```python
from build123d import *

# Parameters (mm, degrees)
SKETCH_1_R          = 8
SKETCH_1_R_2        = 4
EXTRUDE_1_DEPTH     = 7
SKETCH_2_R          = 3
EXTRUDE_2_DEPTH     = 9.5
SKETCH_5_R          = 4
CUT_EXTRUDE_1_DEPTH = 9.5
SKETCH_6_R          = 2
EXTRUDE_3_DEPTH     = 6.5
SKETCH_7_R          = 5.5
CUT_EXTRUDE_2_DEPTH = 2.5


with BuildPart() as part:
    # 草图1 → 凸台-拉伸1 (new body)
    with BuildSketch(Plane(origin=(0, 0, 0), x_dir=(1, 0, 0), z_dir=(0, 1, 0))):
        Circle(SKETCH_1_R)
        Circle(SKETCH_1_R_2, mode=Mode.SUBTRACT)
    extrude(amount=EXTRUDE_1_DEPTH)

    # 草图2 → 凸台-拉伸2 (add)
    with BuildSketch(Plane.XY):
        with Locations((0, 3.5)):
            Circle(SKETCH_2_R)
    extrude(amount=EXTRUDE_2_DEPTH)

    # 草图5 → 切除-拉伸1 (cut)
    with BuildSketch(Plane(origin=(0, 7, 0), x_dir=(1, 0, 0), z_dir=(0, 1, 0))):
        Circle(SKETCH_5_R)
    extrude(amount=-CUT_EXTRUDE_1_DEPTH, mode=Mode.SUBTRACT)

    # 草图6 → 凸台-拉伸3 (add)
    with BuildSketch(Plane.XY.offset(9.5)):
        with Locations((0, 3.5)):
            Circle(SKETCH_6_R)
    extrude(amount=EXTRUDE_3_DEPTH)

    # 草图7 → 切除-拉伸2 (cut)
    with BuildSketch(Plane(origin=(0, 7, 0), x_dir=(1, 0, 0), z_dir=(0, 1, 0))):
        Circle(SKETCH_7_R)
    extrude(amount=-CUT_EXTRUDE_2_DEPTH, mode=Mode.SUBTRACT)


solid = part.part
```
Input: part model. Units: mm. Frame: model coordinates. A direction names the side the tool comes from. Coordinates: 2 decimals unless noted, no trailing zeros. Loops run counter-clockwise (first coordinate to the right, second up) from the corner with the lowest first, then second, coordinate; pieces in that order, holes last. Notation, with made-up numbers: (71, 5) - (129, 5) arc R15 ccw to (129, 24) - close; hole circle Ø2 at (22.5, 84). An arc over 180 degrees is marked (long way). Answer in a Markdown table with one row per item.
(1) Cut plane D-D on z = -4.25. Output: boundary loops of the cut face in (x, y).
Model answer:
| item | result |
|---|---|
| outline | (-6.78, 0) - (6.78, 0) - (6.78, 7) - (3.49, 7) - (3.49, 4.5) - (-3.49, 4.5) - (-3.49, 7) - (-6.78, 7) - close |
(2) Cut plane A-A on z = 0. Output: boundary loops of the cut face in (x, y).
Model answer:
| item | result |
|---|---|
| outline | (-8, 0) - (-4, 0) - (-4, 4.5) - (-5.5, 4.5) - (-5.5, 7) - (-8, 7) - close; (4, 0) - (8, 0) - (8, 7) - (5.5, 7) - (5.5, 4.5) - (4, 4.5) - close |
(3) Cut plane C-C on y = 3.5. Output: boundary loops of the cut face in (x, z).
Model answer:
| item | result |
|---|---|
| outline | (-3, 7.42) arc R8 ccw (long way) to (3, 7.42) - (3, 9.5) - (2, 9.5) - (2, 16) - (-2, 16) - (-2, 9.5) - (-3, 9.5) - close; hole circle Ø8 at (0, 0) |
(4) Set-up query: faces 4 (the face through (1.384, 0.838, 8.675)), 5 (the face through (-4, 4.5, 2)), 6 (the face through (0, 4, 16)). Return all of +Z, -Z, +X, -X, +Y, -Y with unobstructed straight access to the full face (end or side cutting, diameter ignored); none if empty.
Model answer:
| item | result |
|---|---|
| face 4 | +Z |
| face 5 | +Y |
| face 6 | +Z, +X, -X, +Y, -Y |
(5) Mould query, pull axis X, two halves, no side actions, for faces 1 (the face through (1.7, 7, -5.4)), 2 (the face through (-1.19, 5.77, 5.37)), 3 (the face through (4.301, 3.451, -6.746)). Classes: pulls with the +X half, pulls with the -X half, needs draft (parallel to the pull), parting line crosses it, or undercut.
Model answer:
| item | result |
|---|---|
| face 1 | needs draft |
| face 2 | undercut |
| face 3 | parting line crosses it |
(6) Material intervals for L1, parallel to X at y = 5.25, z = 0; L2, parallel to X at y = 1.75, z = 0; L3, parallel to Z at x = 0, y = 1.35, sorted ascending. Write a range as from..to.
Model answer:
| item | result |
|---|---|
| L1 | x = -8..-5.5, 5.5..8 |
| L2 | x = -8..-4, 4..8 |
| L3 | z = -8..-4, 4..9.5 |
(7) Cut plane B-B on x = 0. Output: boundary loops of the cut face in (y, z), plus the area to 3 significant figures.
Model answer:
| item | result |
|---|---|
| outline | (0, -8) - (7, -8) - (7, -5.5) - (4.5, -5.5) - (4.5, -4) - (0, -4) - close; (0, 4) - (4.5, 4) - (4.5, 5.5) - (7, 5.5) - (7, 8) - (6.5, 8) - (6.5, 9.5) - (5.5, 9.5) - (5.5, 16) - (1.5, 16) - (1.5, 9.5) - (0.5, 9.5) - (0.5, 8) - (0, 8) - close |
| area | 83.5 mm² |
(8) Pin query (flat end, axial travel): P1, Ø3.5, axis at x = 0, z = 0.5, coming from the +Y side; P2, Ø2, axis at y = 4, z = 4.5, coming from the +X side; P3, Ø9, axis at x = 0, z = 0, coming from the +Y side; P4, Ø2, axis at x = -3.5, y = 3.5, coming from the -Z side. Return the tip coordinate at first contact, or that it passes through.
Model answer:
| item | result |
|---|---|
| P1 | passes through |
| P2 | stops at x = 7.19 |
| P3 | stops at y = 4.5 |
| P4 | stops at z = -7.6 |
